Input: part model. Units: mm. Frame: model coordinates. A direction names the side the tool comes from. Coordinates: 2 decimals unless noted, no trailing zeros. Write each loop counter-clockwise with the first axis right and the second up, starting at its lowest first coordinate (ties: lowest second). Pieces come first, ordered by that corner, then holes.
1) Section query C-C (y = 2.35). State how many separate pieces and enclosed holes the cut face has, then the cut area to 3 significant figures.
2) Section query B-B (z = -1). Output: boundary loops of the cut face in (x, y) (3 decimals), then the cut area to 3 significant figures.
3) Section query A-A (x = -5.5). Output: boundary loops of the cut face in (y, z) (3 decimals).
4) Line query: L1, parallel to X at y = 0.9, z = -5; L2, parallel to Z at x = 4, y = 0.75; L3, parallel to X at y = 1.6, z = -35. Output: solid intervals per line, ascending.
5) Section query D-D (z = -83). Output: boundary loops of the cut face in (x, y) (3 decimals), then the cut area to 3 significant figures.
6) Draft query along Z for faces 1 (the flat face through (0, 2, 19.05)), 2 (the cylindrical face through (18.204, 1.61, -80.834)), 3 (the flat face through (0, 0, -39)). Return one class per face: pulls with the +Z half, pulls with the -Z half, needs draft (parallel to the pull), parting line crosses it, or undercut.
7) Pin query (flat end, axial travel): pin 1 Ø1.9 at (x, z) = (18.13, -35) entering from -Y; pin 2 Ø1 at (x, y) = (29.5, 1.5) entering from -Z; pin 3 Ø1.6 at (y, z) = (2.5, -53.5) entering from -X. Return the tip coordinate at first contact, or that it passes through.
8) Set-up query: faces 4 (the flat face through (-20.64, 2, 0)), 5 (the flat face through (-26.115, 2, -58)), 6 (the cylindrical face through (33.43, 1.61, -18.45)). Return all of +Z, -Z, +X, -X, +Y, -Y with unobstructed straight access to the full face (end or side cutting, diameter ignored); none if empty.
from build123d import *

# Parameters (mm, degrees)
BOSS_EXTRUDE1_DEPTH = 3.175
SKETCH2_R           = 2.35
SKETCH2_W           = 41
SKETCH2_H           = 21
CUT_EXTRUDE1_DEPTH  = 102.186180504
FILLET1_R           = 2
SKETCH5_R           = 1.5875
CUT_EXTRUDE2_DEPTH  = 102.186180504


with BuildPart() as part:
    # Sketch1 → Boss-Extrude1 (new body)
    with BuildSketch(Plane(origin=(0, 0, 0), x_dir=(1, 0, 0), z_dir=(0, 1, 0))):
        Polygon((-26.115438157, 19.05), (-34, 19.05), (-34, -19.05), (34, -19.05), (34, 19.05), (24.684561843, 19.05), (24.684561843, 95.25), (-26.115438157, 95.25), align=None)
    extrude(amount=BOSS_EXTRUDE1_DEPTH)

    # Sketch2 → Cut-Extrude1 (cut, through all)
    with BuildSketch(Plane(origin=(0, 3.175, 0), x_dir=(1, 0, 0), z_dir=(0, 1, 0))):
        with Locations(Location((-25.640438157, 5, 0), (0, 0, 270))):
            Circle(SKETCH2_R)
        with Locations(Location((-25.640438157, -5, 0), (0, 0, 270))):
            Circle(SKETCH2_R)
        with Locations(Location((25.359561843, -5, 0), (0, 0, 90))):
            Circle(SKETCH2_R)
        with Locations(Location((25.359561843, 5, 0), (0, 0, 90))):
            Circle(SKETCH2_R)
        with Locations((-0.140438157, 0.440263383)):
            Rectangle(SKETCH2_W, SKETCH2_H)
    extrude(amount=-CUT_EXTRUDE1_DEPTH, mode=Mode.SUBTRACT)

    # Fillet1
    fillet1_edges = [part.edges().sort_by_distance(p)[0] for p in [
        (-34, 1.5875, -19.05),
        (34, 1.5875, -19.05),
        (34, 1.5875, 19.05),
        (-34, 1.5875, 19.05),
        (-20.640438157, 1.5875, 10.059736617),
        (-20.640438157, 1.5875, -10.940263383),
        (20.359561843, 1.5875, -10.940263383),
        (20.359561843, 1.5875, 10.059736617),
    ]]
    fillet(fillet1_edges, radius=FILLET1_R)

    # Sketch5 → Cut-Extrude2 (cut, through all)
    with BuildSketch(Plane(origin=(0, 3.175, 0), x_dir=(1, 0, 0), z_dir=(0, 1, 0))):
        with Locations(Location((18.134561843, 79.248, 0), (0, 0, 270))):
            Circle(SKETCH5_R)
        with Locations(Location((18.134561843, 34.998, 0), (0, 0, 270))):
            Circle(SKETCH5_R)
    extrude(amount=-CUT_EXTRUDE2_DEPTH, mode=Mode.SUBTRACT)


solid = part.part
Answer:
1. separate pieces: 1
1. enclosed holes: 7
1. area: 5,520 mm2
2. outline: (-34, 0) - (-20.64, 0) - (-20.64, 3.175) - (-34, 3.175) - close; (20.36, 0) - (34, 0) - (34, 3.175) - (20.36, 3.175) - close
2. area: 85.7 mm2
3. outline: (0, -95.25) - (3.175, -95.25) - (3.175, -10.94) - (0, -10.94) - close; (0, 10.06) - (3.175, 10.06) - (3.175, 19.05) - (0, 19.05) - close
4. L1: x = -34 to -27.99, -23.29 to -20.64, 20.36 to 23.01, 27.71 to 34
4. L2: z = -95.25 to -10.94, 10.06 to 19.05
4. L3: x = -26.12 to 16.55, 19.72 to 24.68
5. outline: (-26.115, 0) - (24.685, 0) - (24.685, 3.175) - (-26.115, 3.175) - close
5. area: 161 mm2
6. face 1: pulls with the +Z half
6. face 2: undercut
6. face 3: needs draft
7. pin 1: passes through
7. pin 2: stops at z = -19.05
7. pin 3: stops at x = -26.12
8. face 4: +Y, -Y
8. face 5: -Z, -X, +Y, -Y
8. face 6: -Z, +X, +Y, -Y
